Here's how the part is built. I have some questions about the finished solid (model axes, mm). A direction names the side the tool comes from. Round coordinates to 2 decimals unless told otherwise and drop trailing zeros. Write each loop counter-clockwise with the first axis right and the second up, starting at its lowest first coordinate (ties: lowest second). Pieces come first, ordered by that corner, then holes. Notation, with made-up numbers: (49, -22.5) - (100, -22.5) arc R28 ccw to (100, -3.5) - close; hole circle Ø7 at (86.5, 22). An arc over 180 degrees is marked (long way). Write item = value, one per line. Start each with the question number.
Item 1: If we section it at C-C (x = 11.15): Please give me the cut outline in (y, z).
Item 2: Which directions (+Z, -Z, +X, -X, +Y, -Y) give clear straight access to the entire face, cutting with the end or side of a thin tool? Please do faces 4 (the face through (44, 12, 11.35)), 5 (the face through (59, 25, 13)), 6 (the face through (14.68, 2.96, -1.11)).
Item 3: If we section it at D-D (x = 20.5): Please give me the cut outline in (y, z).
Item 4: Thinking about a two-plate mould opening in Y: for faces 1 (the face through (62.668, 16.314, 5.779)), 2 (the face through (44, 12, -11.35)), 3 (the face through (31, 6, 0)), which applies, pulls with the +Y half, pulls with the -Y half, needs draft (parallel to the pull), parting line crosses it, or undercut?
Item 5: If we section it at A-A (z = 6): Please give me the cut outline in (x, y), and give its area (3 significant figures).
Item 6: For P1, Ø1.5, axis at y = 25.5, z = 9.5, coming from the -X side; P2, Ø1.4, axis at y = 25, z = 12, coming from the -X side; P3, Ø6, axis at x = 50.85, z = 0, coming from the +Y side, each with a flat end and sliding along its axis, tell me the tip position at first contact or that it passes through.
Item 7: If I drill on line 1 along X through (y, z) = (3.7, 0); line 2 along Y through (x, z) = (63.8, 0); line 3 along Y through (x, z) = (63.6, 6), over which ranges is the centre line in solid material (lowest first)? Write a range as [from, to].
Item 8: If we section it at B-B (y = 18): Please give me the cut outline in (x, z).
```python
from build123d import *

# Parameters (mm, degrees)
EXTRUDE_1_DEPTH     = 14.15
SKETCH_2_W          = 60.4
SKETCH_2_H          = 24
CUT_EXTRUDE_1_DEPTH = 11.35
CUT_EXTRUDE_2_REACH = 74.974
SKETCH_4_R          = 2.55
SKETCH_4_R_2        = 3.7
CUT_EXTRUDE_3_REACH = 74.974
SKETCH_5_R          = 1.7


with BuildPart() as part:
    # 草图1 → 凸台-拉伸1 (new, symmetric)
    with BuildSketch(Plane.XY):
        Polygon((0, 0), (65, 0), (65, 30), (59, 30), (59, 20), (10, 6), (0, 6), align=None)
    extrude(amount=EXTRUDE_1_DEPTH, both=True)

    # 草图2 → 切除-拉伸1 (cut, symmetric)
    with BuildSketch(Plane.XY):
        with Locations((30.2, 18)):
            Rectangle(SKETCH_2_W, SKETCH_2_H)
    extrude(amount=CUT_EXTRUDE_1_DEPTH, both=True, mode=Mode.SUBTRACT)

    # 草图4 → 切除-拉伸2 (cut, up to next)
    with BuildSketch(Plane(origin=(0, 0, 0), x_dir=(1, 0, 0), z_dir=(0, 1, 0)), mode=Mode.PRIVATE) as cut_extrude_2_sk1:
        with Locations((50.85, 0)):
            Circle(SKETCH_4_R)
    cut_extrude_2_tool1 = extrude(cut_extrude_2_sk1.sketch, amount=CUT_EXTRUDE_2_REACH, mode=Mode.PRIVATE) & part.part
    # 草图4 → 切除-拉伸2 (cut, up to next)
    with BuildSketch(Plane(origin=(0, 0, 0), x_dir=(1, 0, 0), z_dir=(0, 1, 0)), mode=Mode.PRIVATE) as cut_extrude_2_sk2:
        with Locations((11.15, 0)):
            Circle(SKETCH_4_R_2)
    cut_extrude_2_tool2 = extrude(cut_extrude_2_sk2.sketch, amount=CUT_EXTRUDE_2_REACH, mode=Mode.PRIVATE) & part.part
    add(cut_extrude_2_tool1.solids().sort_by_distance((50.85, 0, 0))[0], mode=Mode.SUBTRACT)
    add(cut_extrude_2_tool2.solids().sort_by_distance((11.15, 0, 0))[0], mode=Mode.SUBTRACT)

    # 草图5 → 切除-拉伸3 (cut, up to next)
    with BuildSketch(Plane(origin=(0, 0, 0), x_dir=(0, 0, -1), z_dir=(1, 0, 0)), mode=Mode.PRIVATE) as cut_extrude_3_sk1:
        with Locations(Location((0, 24, 0), (0, 0, 180))):
            Circle(SKETCH_5_R)
    cut_extrude_3_tool1 = extrude(cut_extrude_3_sk1.sketch, amount=CUT_EXTRUDE_3_REACH, mode=Mode.PRIVATE) & part.part
    # 草图5 → 切除-拉伸3 (cut, up to next)
    with BuildSketch(Plane(origin=(0, 0, 0), x_dir=(0, 0, -1), z_dir=(1, 0, 0)), mode=Mode.PRIVATE) as cut_extrude_3_sk2:
        with Locations(Location((0, 12, 0), (0, 0, 180))):
            Circle(SKETCH_5_R)
    cut_extrude_3_tool2 = extrude(cut_extrude_3_sk2.sketch, amount=CUT_EXTRUDE_3_REACH, mode=Mode.PRIVATE) & part.part
    # 草图5 → 切除-拉伸3 (cut, up to next)
    with BuildSketch(Plane(origin=(0, 0, 0), x_dir=(0, 0, -1), z_dir=(1, 0, 0)), mode=Mode.PRIVATE) as cut_extrude_3_sk3:
        with Locations(Location((-6, 18, 0), (0, 0, 180))):
            Circle(SKETCH_5_R)
    cut_extrude_3_tool3 = extrude(cut_extrude_3_sk3.sketch, amount=CUT_EXTRUDE_3_REACH, mode=Mode.PRIVATE) & part.part
    # 草图5 → 切除-拉伸3 (cut, up to next)
    with BuildSketch(Plane(origin=(0, 0, 0), x_dir=(0, 0, -1), z_dir=(1, 0, 0)), mode=Mode.PRIVATE) as cut_extrude_3_sk4:
        with Locations(Location((6, 18, 0), (0, 0, 180))):
            Circle(SKETCH_5_R)
    cut_extrude_3_tool4 = extrude(cut_extrude_3_sk4.sketch, amount=CUT_EXTRUDE_3_REACH, mode=Mode.PRIVATE) & part.part
    add(cut_extrude_3_tool1.solids().sort_by_distance((0, 24, 0))[0], mode=Mode.SUBTRACT)
    add(cut_extrude_3_tool2.solids().sort_by_distance((0, 12, 0))[0], mode=Mode.SUBTRACT)
    add(cut_extrude_3_tool3.solids().sort_by_distance((0, 18, 6))[0], mode=Mode.SUBTRACT)
    add(cut_extrude_3_tool4.solids().sort_by_distance((0, 18, -6))[0], mode=Mode.SUBTRACT)


solid = part.part
```
Reply:
q1.outline = (0, -14.15) - (6.33, -14.15) - (6.33, -11.35) - (6, -11.35) - (6, -3.7) - (0, -3.7) - close; (0, 3.7) - (6, 3.7) - (6, 11.35) - (6.33, 11.35) - (6.33, 14.15) - (0, 14.15) - close
q2.face_4 = -X, +Y
q2.face_5 = +Z, -Z, -X, +Y
q2.face_6 = +Y, -Y
q3.outline = (0, -14.15) - (9, -14.15) - (9, -11.35) - (6, -11.35) - (6, 11.35) - (9, 11.35) - (9, 14.15) - (0, 14.15) - close
q4.face_1 = undercut
q4.face_2 = needs draft
q4.face_3 = pulls with the +Y half
q5.outline = (0, 0) - (65, 0) - (65, 16.3) - (60.4, 16.3) - (60.4, 6) - (0, 6) - close; (60.4, 19.7) - (65, 19.7) - (65, 30) - (60.4, 30) - close
q5.area = 485 mm2
q6.P1 = 60.4
q6.P2 = 59
q6.P3 = 6
q7.line_1 = [0, 7.45], [14.85, 48.3], [53.4, 65]
q7.line_2 = [0, 10.3], [13.7, 22.3], [25.7, 30]
q7.line_3 = [0, 16.3], [19.7, 30]
q8.outline = (52, -14.15) - (65, -14.15) - (65, -7.7) - (60.4, -7.7) - (60.4, -11.35) - (52, -11.35) - close; (52, 11.35) - (60.4, 11.35) - (60.4, 7.7) - (65, 7.7) - (65, 14.15) - (52, 14.15) - close; (60.4, -4.3) - (65, -4.3) - (65, 4.3) - (60.4, 4.3) - close
